The model under review builds one solid part; all positions refer to its coordinate system, in mm. Face numbers are marked on the shaded views. A direction names the side the tool comes from. Round coordinates to 2 decimals unless told otherwise and drop trailing zeros. Order: outer loops, then holes, each group sorted by start corner. A loop starts at its lowest first (then second) coordinate and runs counter-clockwise, first axis right, second up. Notation, with made-up numbers: M 13,28 L 64,28 A17 cw 64,36 Z; hole C 77.25,52.25 d4. An arc over 180 degrees is marked long. Answer as a JSON object with one key per item and string values. Group by question number.
1. Add section B-B on y = -482.6. State the section outline as (x, z) points, and give its area (3 significant figures).
2. Mouldability with a two-part tool opening along Y and no side actions: class the marked faces 3, 4 and 5 as released by +Y, released by -Y, zero draft, split by the parting line, or undercut.
3. Add section D-D on z = 429. State the section outline as (x, y) points.
4. Clearance check with flat-ended pins moving along their axes: P1, Ø10, axis at x = -143, y = -616, coming from the +Z side; P2, Ø13.5, axis at x = -334, z = 509.5, coming from the -Y side; P3, Ø1.9, axis at x = -78, y = -611.5, coming from the -Z side; P4, Ø4, axis at y = -103.5, z = 509, coming from the +X side. State where each tip first meets the part, or that it passes through.
5. Add section C-C on y = -378.5. State the section outline as (x, z) points, and give its area (3 significant figures).
6. To check wall thickness, follow probe 1 along Z at (x, y) = (-230.5, -426.5); probe 2 along Y at (x, z) = (-278.5, 166.5); probe 3 along Y at (x, z) = (-98, -230). State the ranges of each line that lie inside material, in increasing order. Write a range as [from, to].
7. Machinability: for the marked faces 1 and 2, which of the approach directions +Z, -Z, +X, -X, +Y, -Y give a long, thin tool a straight path to every point of the face, cutting with its end or side? Answer none if there is none.
8. Add section A-A on z = -167. State the section outline as (x, y) points.
```python
from build123d import *

# Parameters (mm, degrees)
F0_W      = 609.6
F0_H      = 863.6
F1_DEPTH  = 609.6
F2_W      = 609.6
F2_H      = 101.6
F3_DEPTH  = 127
F4_R      = 88.9
F4_R_2    = 63.5
F5_DEPTH  = 6.35
F6_W      = 558.8
F6_H      = 254
F7_DEPTH  = 6.35
F8_W      = 609.6
F8_H      = 495.3
F8_H_2    = 44.45
F9_DEPTH  = 12.7
F10_W     = 457.2
F10_H     = 25.4
F11_DEPTH = 12.7
F12_W     = 152.4
F12_H     = 50.8
F13_DEPTH = 5.08
F14_R     = 22.225
F15_DEPTH = 25.4


with BuildPart() as f1:
    # F0 (on Front) → F1 (new body)
    with BuildSketch(Plane.XZ):
        with Locations((-87.74905, 10.130912)):
            Rectangle(F0_W, F0_H)
    extrude(amount=F1_DEPTH)

    # F2 (on face) → F3 (join)
    with BuildSketch(Plane.XY.offset(441.930912)):
        with Locations((-87.74905, -50.8)):
            Rectangle(F2_W, F2_H)
    extrude(amount=F3_DEPTH)

    # F4 (on face) → F5 (join)
    with BuildSketch(Plane.XY.offset(441.930912)):
        with Locations((-214.74905, -228.6)):
            Circle(F4_R)
        with Locations((-214.74905, -482.6)):
            Circle(F4_R_2)
        with Locations((39.25095, -482.6)):
            Circle(F4_R)
        with Locations((39.25095, -228.6)):
            Circle(F4_R_2)
    extrude(amount=F5_DEPTH)

    # F6 (on face) → F7 (join)
    with BuildSketch(Plane.XZ.offset(609.6)):
        with Locations((-87.74905, -269.269088)):
            Rectangle(F6_W, F6_H)
    extrude(amount=F7_DEPTH)

    # F8 (on face) → F9 (join)
    with BuildSketch(Plane.XZ.offset(609.6)):
        with Locations((-87.74905, 143.480912)):
            Rectangle(F8_W, F8_H)
        with Locations((-87.74905, 419.705912)):
            Rectangle(F8_W, F8_H_2)
    extrude(amount=F9_DEPTH)

    # F10 (on face) → F11 (join)
    with BuildSketch(Plane.XZ.offset(622.3)):
        with Locations((-87.74905, 352.542192)):
            Rectangle(F10_W, F10_H)
    extrude(amount=F11_DEPTH)

    # F12 (on face) → F13 (join)
    with BuildSketch(Plane.XZ.offset(101.6)):
        with Locations((-87.74905, 505.430912)):
            Rectangle(F12_W, F12_H)
    extrude(amount=F13_DEPTH)

    # F14 (on face) → F15 (join)
    with BuildSketch(Plane.XZ.offset(101.6)):
        with Locations((-329.04905, 505.430912)):
            Circle(F14_R)
        with Locations((-252.84905, 505.430912)):
            Circle(F14_R)
        with Locations((77.35095, 505.430912)):
            Circle(F14_R)
        with Locations((153.55095, 505.430912)):
            Circle(F14_R)
    extrude(amount=F15_DEPTH)


solid = f1.part
```
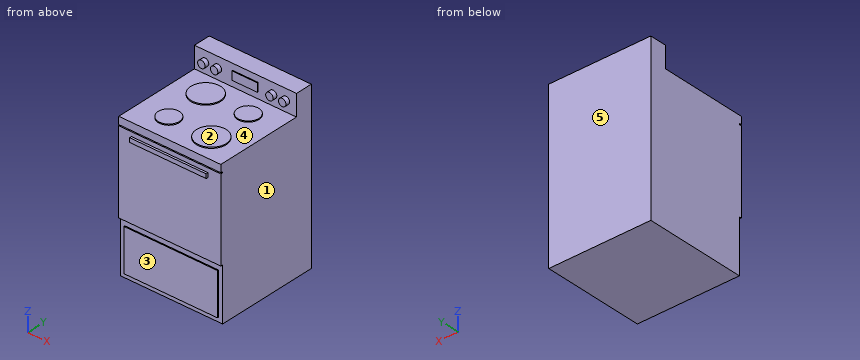
Recorded:
{
 "1": {"outline": "M -392.55,-421.67 L 217.05,-421.67 L 217.05,441.93 L 128.15,441.93 L 128.15,448.28 L -49.65,448.28 L -49.65,441.93 L -151.25,441.93 L -151.25,448.28 L -278.25,448.28 L -278.25,441.93 L -392.55,441.93 Z", "area": "528,000 mm²"},
 "2": {"face 3": "released by -Y", "face 4": "undercut", "face 5": "released by +Y"},
 "3": {"outline": "M -392.55,-622.3 L 217.05,-622.3 L 217.05,0 L -392.55,0 Z"},
 "4": {"P1": "stops at z = 441.93", "P2": "stops at y = -127", "P3": "stops at z = -396.27", "P4": "stops at x = 217.05"},
 "5": {"outline": "M -392.55,-421.67 L 217.05,-421.67 L 217.05,441.93 L -392.55,441.93 Z", "area": "526,000 mm²"},
 "6": {"probe 1": "z = [-421.67, 448.28]", "probe 2": "y = [-622.3, 0]", "probe 3": "y = [-615.95, 0]"},
 "7": {"face 1": "+Z, -Z, +X, +Y, -Y", "face 2": "+Z, +X, -X, -Y"},
 "8": {"outline": "M -392.55,-609.6 L -367.15,-609.6 L -367.15,-615.95 L 191.65,-615.95 L 191.65,-609.6 L 217.05,-609.6 L 217.05,0 L -392.55,0 Z"}
}
